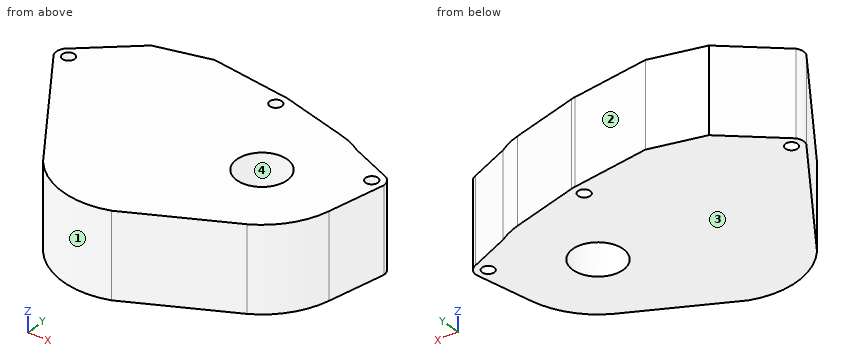
Autodesk Inventor part; units mm, degrees
ref_plane "YZ Plane" through (0, 0, 0) normal (1, 0, 0) x (0, 1, 0)
ref_plane "XZ Plane" through (0, 0, 0) normal (0, 1, 0) x (-1, 0, 0)
ref_plane "XY Plane" through (0, 0, 0) normal (0, 0, 1) x (1, 0, 0)
sketch "Sketch1" plane through (0, 0, 0) normal (0, 0, 1) x (1, 0, 0)
  circle A0 centre (0, 0) radius 3
  circle A1 centre (149.4, 0) radius 3
  circle A2 centre (85.7991, 21.6971) radius 3
  circle A3 centre (110.2989, -19.8991) radius 12.5
  arc A4 (87.814, 27.3487) -> (83.7842, 27.3487) centre (85.7991, 21.6971) ccw
  arc A5 (154.885, -2.4321) -> (151.3594, 5.6711) centre (149.4, 0) ccw
  arc A6 (-0.9713, 5.9209) -> (-1.9594, -5.6711) centre (0, 0) ccw
  line L0 (-1.9594, 5.6711) -> (-0.9713, 5.9209)
  line L1 (87.814, 27.3487) -> (120.8026, 18.6971)
  line L2 (131.5219, 14.0064) -> (151.3594, 5.6711)
  line L3 (155.4, 0) -> (149.4311, -28.1861)
  arc A7 (131.5219, 14.0064) -> (120.0887, 18.8843) centre (110.2989, -19.8991) ccw
  line L4 (21.1662, 25.9822) -> (47.4365, 32.6255)
  line L5 (-4.9033, 3.458) -> (21.1662, 25.9822)
  line L6 (85.7991, 27.6971) -> (47.4365, 32.6255)
  line L7 (0, 0) -> (2.9084, 0.7355)
  line L8 (82.8907, 20.9616) -> (85.7991, 21.6971)
  arc A8 (125.9738, -56.7) -> (149.4311, -28.1861) centre (110.2989, -19.8991) ccw
  line L9 (80.7723, -79.2884) -> (129.3991, -55.0443)
  line L10 (-4.37, -4.1113) -> (37.9799, -67.1663)
  arc A9 (88.5511, 22.8914) -> (86.7834, 21.946) centre (110.2989, -19.8991) ccw
  arc A10 (154.9491, -2.282) -> (150.7621, 5.922) centre (110.2989, -19.8991) ccw
  arc A11 (33.9775, -61.2072) -> (80.7723, -79.2884) centre (68.0362, -42.6558) ccw
  point P0 (111.3369, -59.8857)
  dimension "d3" = 6
  dimension "d5" = 6
  dimension "d15" = 6
  dimension "d18" = 25
  dimension "d19" = 12
  dimension "d20" = 12
  dimension "d21" = 12
extrude "Extrusion2" add sketch "Sketch1" along normal blind 42 contours L1 A7 L2 A10 L3 A8 L9 A11 L10 A6 L5 L4 L6 A4 | L2 A5 L3 A10
properties part number "body droit"
Design review of the part built by this model. Coordinates are the model's own, in mm. Face numbers are marked on the shaded views. Round coordinates to 2 decimals unless told otherwise and drop trailing zeros. Order: outer loops, then holes, each group sorted by start corner. A loop starts at its lowest first (then second) coordinate and runs counter-clockwise, first axis right, second up.
1) Consider section C-C (x = 33.5). State the section outline as (y, z) points.
The answers:
outline: (-60.5, 0) - (29.1, 0) - (29.1, 42) - (-60.5, 42) - close
2) Consider section A-A (y = -22.5). State the section outline as (x, z) points, plus the area to 3 significant figures.
The answers:
outline: (7.98, 0) - (98.07, 0) - (98.07, 42) - (7.98, 42) - close; (122.53, 0) - (150.64, 0) - (150.64, 42) - (122.53, 42) - close
area: 4,960 mm2
3) Consider section D-D (y = -37.5). State the section outline as (x, z) points (3 decimals).
The answers:
outline: (18.055, 0) - (146.218, 0) - (146.218, 42) - (18.055, 42) - close
4) For L1, parallel to X at y = -27, z = 10; L2, parallel to Y at x = 0, z = 28.5; L3, parallel to Y at x = 100, z = 19, list the stretches that pass through material, from the lowest coordinate up.
The answers:
L1: x = 11 to 100.01, 120.59 to 149.68
L2: y = -10.62 to -3, 3 to 7.69
L3: y = -69.7 to -26.98, -12.82 to 24.15
5) Consider section B-B (z = 14). State the section outline as (x, y) points.
The answers:
outline: (-4.9, 3.46) arc R6 ccw to (-4.37, -4.11) - (37.98, -67.17) arc R38.78 ccw to (80.77, -79.29) - (129.4, -55.04) arc R40 ccw to (149.43, -28.19) - (155.4, 0) arc R6 ccw to (151.36, 5.67) - (131.52, 14.01) arc R40 ccw to (120.8, 18.7) - (87.81, 27.35) arc R6 ccw to (85.8, 27.7) - (47.44, 32.63) - (21.17, 25.98) - close; hole circle Ø6 at (0, 0); hole (-1.96, 5.67) - (-0.97, 5.92) arc R6 ccw to start; hole circle Ø6 at (85.8, 21.7); hole circle Ø25 at (110.3, -19.9); hole circle Ø6 at (149.4, 0)
6) Draft analysis for pull direction Y (two halves, no side actions). For the marked faces 1, 2, 3 and 4, state which applies: released by +Y, released by -Y, zero draft, split by the parting line, or undercut.
The answers:
face 1: released by -Y
face 2: released by +Y
face 3: zero draft
face 4: undercut
7) Clearance check with flat-ended pins moving along their axes: pin 1 Ø1 at (y, z) = (5, 16) entering from +X; pin 2 Ø1 at (y, z) = (-55.5, 14) entering from +X; pin 3 Ø3.5 at (x, y) = (149.4, 0) entering from +Z; pin 4 Ø12 at (x, z) = (118.5, 32.5) entering from -Y. State where each tip first meets the part, or that it passes through.
The answers:
pin 1: stops at x = 153.37
pin 2: stops at x = 129.48
pin 3: passes through
pin 4: stops at y = -63.47
